The drawing under review shows one solid part. Ordinate dimensions are in mm from its lowest x, y, z. A direction names the side the tool comes from. Coordinates: 2 decimals unless noted, no trailing zeros. Write each loop counter-clockwise with the first axis right and the second up, starting at its lowest first coordinate (ties: lowest second). Pieces come first, ordered by that corner, then holes. Notation, with made-up numbers: M -1.75,88 L 49.25,88 A32 cw 49.25,114 Z; hole C 86,-16 d5. An arc over 180 degrees is marked long. Write each question's results on one line, items separated by ' | '. Start each with the question number.
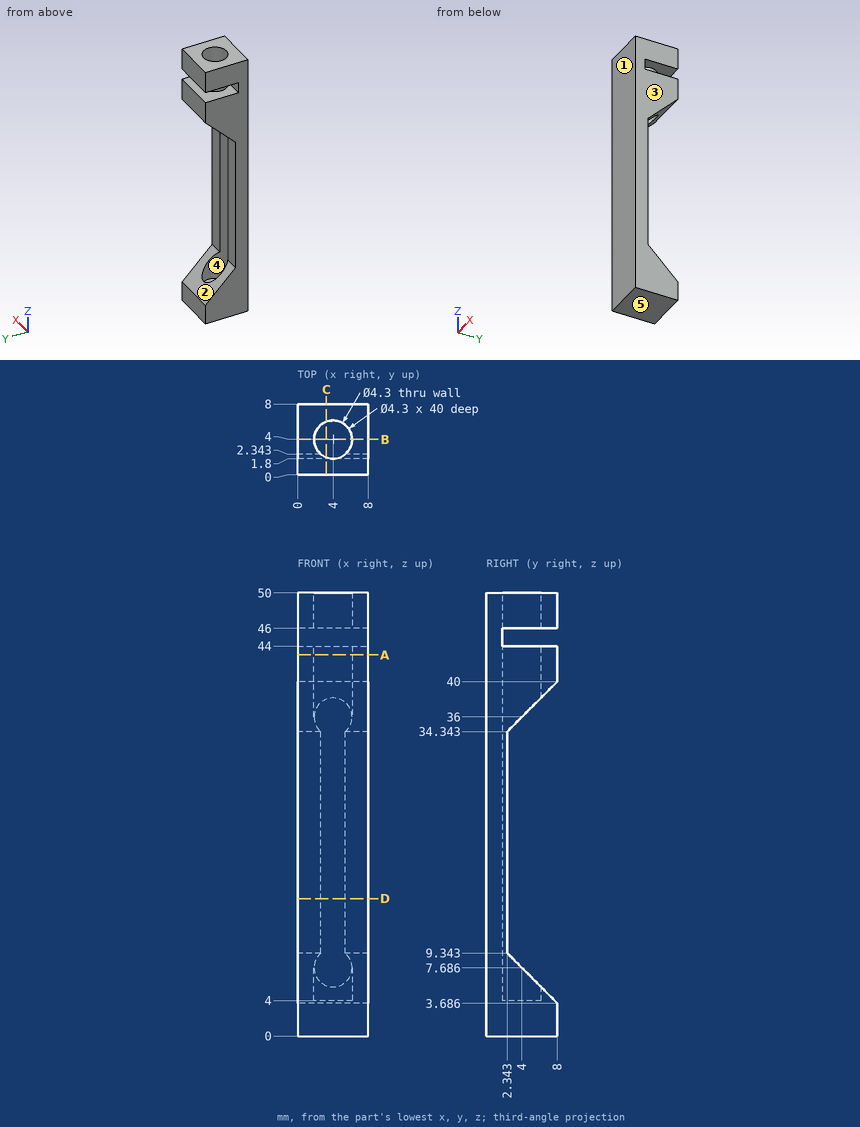
Item 1: Insertion check: pin 1 Ø1 at (x, z) = (5, 30) entering from -Y; pin 2 Ø1 at (x, z) = (7, 11) entering from +Y; pin 3 Ø1 at (x, z) = (3.5, 45) entering from +Y; pin 4 Ø1.3 at (x, y) = (3.5, 5) entering from +Z. Each pin has a flat end and moves straight along its axis. Give the tip position at first contact, or say it passes through.
Item 2: We need section D-D on z = 15.5. State the section outline as (x, y) points, then the cut area to 3 significant figures.
Item 3: We need section A-A on z = 43. State the section outline as (x, y) points.
Item 4: Wall thickness on L1, parallel to Z at x = 6.25, y = 7.5 (1 decimal); L2, parallel to Z at x = 7.5, y = 7 (1 decimal); L3, parallel to Z at x = 5, y = 2: over which ranges is each line inside the solid? List them lowest first.
Item 5: We need section C-C on x = 3.25. Count the separate pieces of the cut face and the enclosed holes in it, then the cut area to 3 significant figures.
Item 6: Draft analysis for pull direction X (two halves, no side actions). For the marked faces 3, 4 and 5, state which applies: released by +X, released by -X, zero draft, split by the parting line, or undercut.
Item 7: We need section B-B on y = 4. State the section outline as (x, z) points.
Item 8: For the marked faces 1 and 2, list the 3-axis set-ups (+Z, -Z, +X, -X, +Y, -Y) from which the entire face can be reached by the end or side of a thin tool; tool diameter is ignored.
Answer:
1) pin 1: stops at y = 0 | pin 2: stops at y = 2.34 | pin 3: stops at y = 1.8 | pin 4: stops at z = 4
2) outline: M 0,0 L 8,0 L 8,2.34 L 5.37,2.34 A2.15 cw 2.63,2.34 L 0,2.34 Z | area: 17.8 mm^2
3) outline: M 0,0 L 8,0 L 8,8 L 0,8 Z; hole C 4,4 d4.3
4) L1: z = 0 to 4.2, 39.5 to 44, 46 to 50 | L2: z = 0 to 4.7, 39 to 44, 46 to 50 | L3: z = 0 to 44, 46 to 50
5) separate pieces: 3 | enclosed holes: 0 | area: 142 mm^2
6) face 3: released by +X | face 4: undercut | face 5: zero draft
7) outline: M 0,0 L 8,0 L 8,7.69 L 6.15,7.69 L 6.15,4 L 1.85,4 L 1.85,7.69 L 0,7.69 Z; M 0,36 L 1.85,36 L 1.85,44 L 0,44 Z; M 0,46 L 1.85,46 L 1.85,50 L 0,50 Z; M 6.15,36 L 8,36 L 8,44 L 6.15,44 Z; M 6.15,46 L 8,46 L 8,50 L 6.15,50 Z
8) face 1: +Z, -Z, +X, -X, -Y | face 2: +X, -X, +Y
